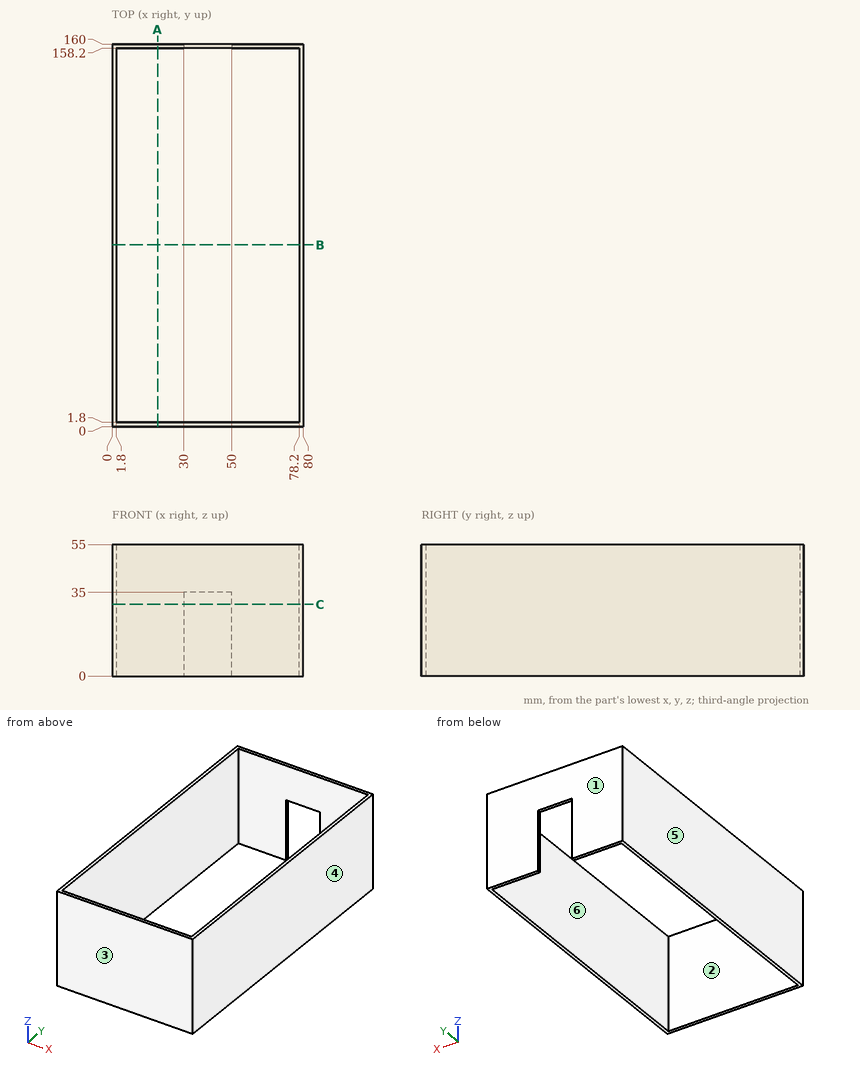
Geometry check sheet. Reference: drawing and pictorial views, mm from the part's lowest x, y, z. A direction names the side the tool comes from. Round coordinates to 2 decimals unless told otherwise and drop trailing zeros. Loops run counter-clockwise (first coordinate to the right, second up) from the corner with the lowest first, then second, coordinate; pieces in that order, holes last. Notation, with made-up numbers: M 57,-36 L 71,-36 A27 cw 71,0 Z; hole C 23.5,83 d11. An arc over 180 degrees is marked long. One line per item, written item: value.
(1) Sectioned sample at C-C, the plane z = 30. Record the cut outline in (x, y), then the cut area to 3 significant figures.
Computed values:
outline: M 0,0 L 80,0 L 80,160 L 50,160 L 50,158.2 L 78.2,158.2 L 78.2,1.8 L 1.8,1.8 L 1.8,158.2 L 30,158.2 L 30,160 L 0,160 Z
area: 815 mm^2
(2) Sectioned sample at B-B, the plane y = 76. Record the cut outline in (x, z), then the cut area to 3 significant figures.
Computed values:
outline: M 0,0 L 1.8,0 L 1.8,55 L 0,55 Z; M 78.2,0 L 80,0 L 80,55 L 78.2,55 Z
area: 198 mm^2
(3) Sectioned sample at A-A, the plane x = 19. Record the cut outline in (y, z).
Computed values:
outline: M 0,0 L 1.8,0 L 1.8,55 L 0,55 Z; M 158.2,0 L 160,0 L 160,55 L 158.2,55 Z
(4) Thickness scan on line 1 (Y direction, x = 74, z = 20.5); line 2 (X direction, y = 151, z = 30.5); line 3 (Y direction, x = 49, z = 7). Record the ranges inside material, lowest first.
Computed values:
line 1: y = 0 to 1.8, 158.2 to 160
line 2: x = 0 to 1.8, 78.2 to 80
line 3: y = 0 to 1.8
(5) Release check for a two-part mould opening along Y. For the marked faces 1, 2, 3 and 4 record: +Y half, -Y half, draft (parallel to the pull), parting line (faces both ways), or undercut.
Computed values:
face 1: +Y half
face 2: undercut
face 3: -Y half
face 4: draft
(6) Depth check by flat-ended pin: pin 1 Ø12 at (x, y) = (69.5, 95.5) entering from -Z; pin 2 Ø0.9 at (x, y) = (39, 159) entering from -Z. Enter the tip coordinate at first touch or a pass-through.
Computed values:
pin 1: passes through
pin 2: stops at z = 35
(7) Access from +Z, -Z, +X, -X, +Y, -Y to the whole of each face (thin tool, end or side, straight path). Record for the marked faces 5 and 6.
Computed values:
face 5: +Z, -Z, -X, +Y, -Y
face 6: +Z, -Z
